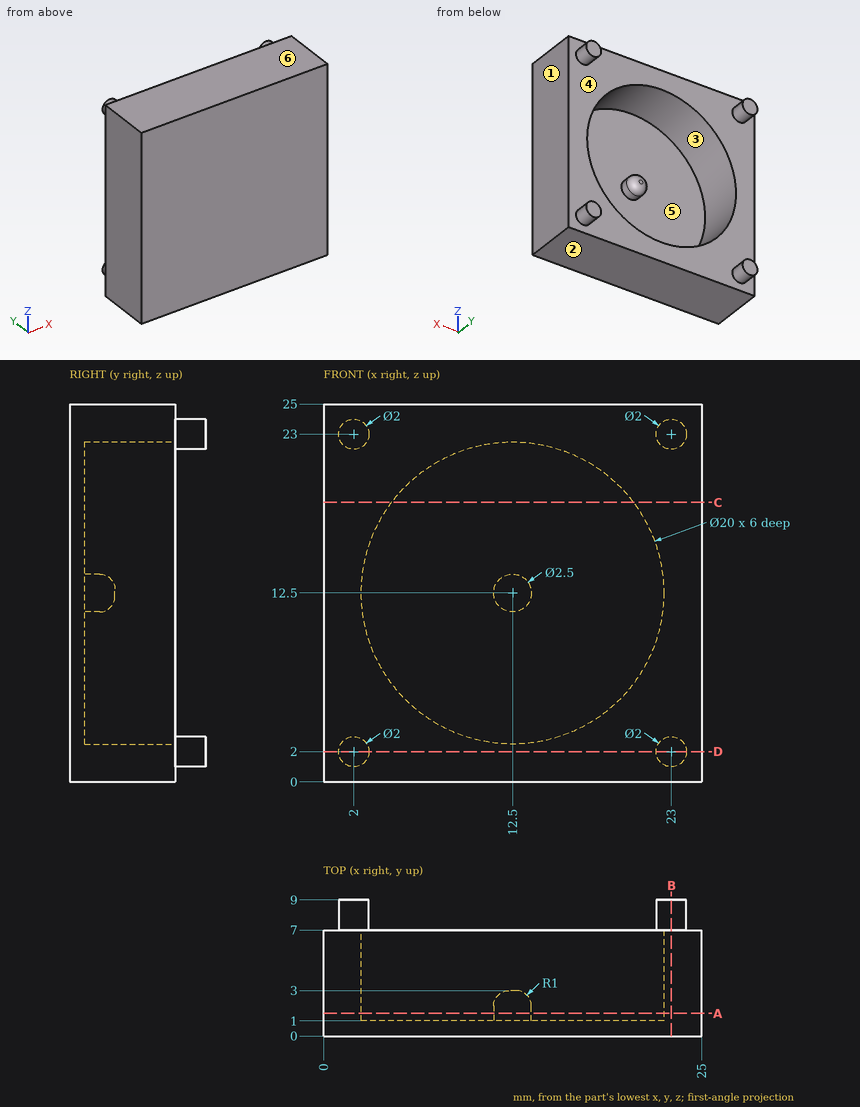
Here's the drawing with two shaded views (mm, measured from the low corner). I have some questions. A direction names the side the tool comes from. Give positions to 0.01 mm unless a question says otherwise; leave off trailing zeros. Loops run counter-clockwise (first coordinate to the right, second up) from the corner with the lowest first, then second, coordinate; pieces in that order, holes last. Notation, with made-up numbers: (5, 13) -> (57, 13) arc R26 ccw to (57, 37) -> close; hole circle Ø8 at (41.25, 48). An arc over 180 degrees is marked (long way). One line per item, written item: value.
Q1. We'd pull the mould along Z, two halves only. Please class the marked faces 1, 2, 3 and 4: pulls with the +Z half, pulls with the -Z half, needs draft (parallel to the pull), parting line crosses it, or undercut.
Answers follow:
face 1: needs draft
face 2: pulls with the -Z half
face 3: undercut
face 4: undercut
Q2. Suppose I cut it at C-C on z = 18.5. Please give me the cut outline in (x, y).
Answers follow:
outline: (0, 0) -> (25, 0) -> (25, 7) -> (20.5, 7) -> (20.5, 1) -> (4.5, 1) -> (4.5, 7) -> (0, 7) -> close
Q3. If I drill on line 1 along X through (y, z) = (4.05, 12.5); line 2 along Z through (x, y) = (12.5, 2.75), over which ranges is the centre line in solid material (lowest first)?
Answers follow:
line 1: 0 to 2.5, 22.5 to 25
line 2: 0 to 2.5, 11.59 to 13.41, 22.5 to 25
Q4. Suppose I cut it at A-A on y = 1.5. Please give me the cut outline in (x, z), then the cut area to 3 significant figures.
Answers follow:
outline: (0, 0) -> (25, 0) -> (25, 25) -> (0, 25) -> close; circle Ø2.5 at (12.5, 12.5); hole circle Ø20 at (12.5, 12.5)
area: 316 mm^2
Q5. On a 3-axis mill with a long thin cutter (end or side, diameter ignored), from which of +Z, -Z, +X, -X, +Y, -Y can I reach the whole of each face in a straight line? I mean the marked faces 5 and 6. Say none if no direction works.
Answers follow:
face 5: +Y
face 6: +Z, +X, -X, +Y, -Y
Q6. I'm going to push a flat-ended pin straight in: pin 1 Ø6 at (x, z) = (10, 12) entering from +Y. Where does the tip first touch, or does it pass through?
Answers follow:
pin 1: y = 3
Q7. Suppose I cut it at B-B on x = 23. Please give me the cut outline in (y, z).
Answers follow:
outline: (0, 0) -> (7, 0) -> (7, 1) -> (9, 1) -> (9, 3) -> (7, 3) -> (7, 22) -> (9, 22) -> (9, 24) -> (7, 24) -> (7, 25) -> (0, 25) -> close
Q8. Suppose I cut it at D-D on z = 2. Please give me the cut outline in (x, y).
Answers follow:
outline: (0, 0) -> (25, 0) -> (25, 7) -> (24, 7) -> (24, 9) -> (22, 9) -> (22, 7) -> (3, 7) -> (3, 9) -> (1, 9) -> (1, 7) -> (0, 7) -> close
